The drawing under review shows one solid part. Ordinate dimensions are in mm from its lowest x, y, z. Coordinates: 2 decimals unless noted, no trailing zeros. Write each loop counter-clockwise with the first axis right and the second up, starting at its lowest first coordinate (ties: lowest second). Pieces come first, ordered by that corner, then holes.
Q1. Add section B-B, the plane z = 0.3. Give the number of separate pieces and of enclosed holes in the cut face, plus the area to 3 significant figures.
Q2. To check wall thickness, follow probe 1 along Y at (x, z) = (40, 0.2); probe 2 along Y at (x, z) = (34, 0.85) (1 decimal); probe 3 along X at (y, z) = (15, 0.5) (1 decimal). State the ranges of each line that lie inside material, in increasing order.
Q3. Add section A-A, the plane y = 40. Give the boundary of the cut face in (x, z).
Q4. Add section D-D, the plane y = 62.5. Give the boundary of the cut face in (x, z).
Q5. Add section C-C, the plane x = 40. Give the boundary of the cut face in (y, z).
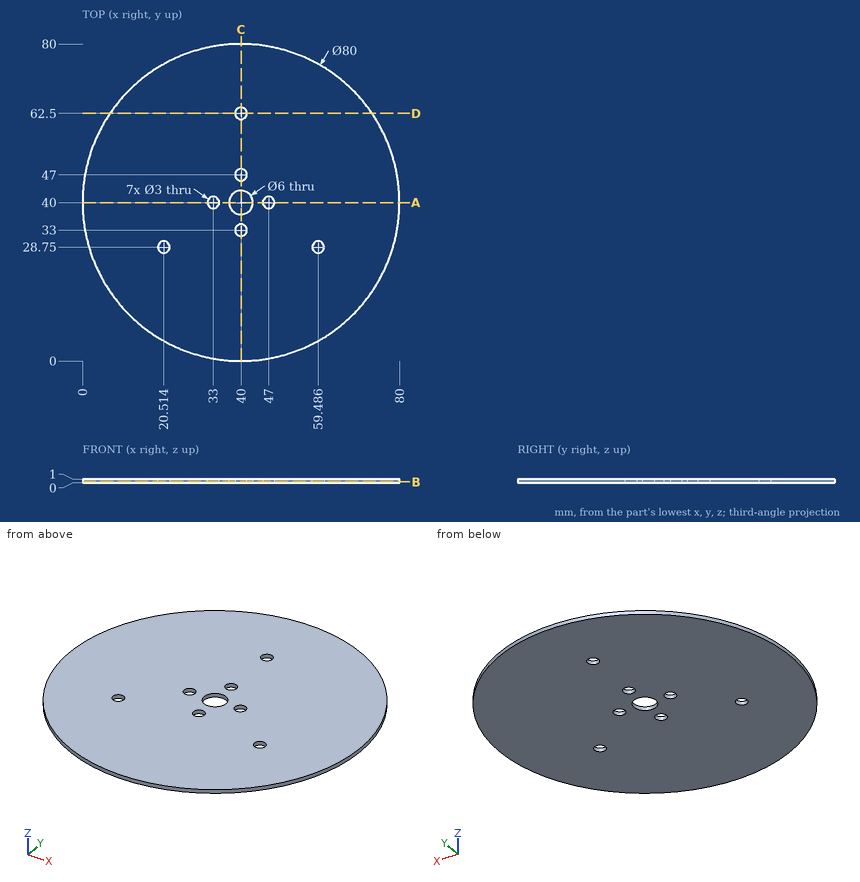
Here are the results:
1. separate pieces: 1
1. enclosed holes: 8
1. area: 4,950 mm2
2. probe 1: y = 0 to 31.5, 34.5 to 37, 43 to 45.5, 48.5 to 61, 64 to 80
2. probe 2: y = 0.5 to 38.9, 41.1 to 79.5
2. probe 3: x = 8.8 to 71.2
3. outline: (0, 0) - (31.5, 0) - (31.5, 1) - (0, 1) - close; (34.5, 0) - (37, 0) - (37, 1) - (34.5, 1) - close; (43, 0) - (45.5, 0) - (45.5, 1) - (43, 1) - close; (48.5, 0) - (80, 0) - (80, 1) - (48.5, 1) - close
4. outline: (6.93, 0) - (38.5, 0) - (38.5, 1) - (6.93, 1) - close; (41.5, 0) - (73.07, 0) - (73.07, 1) - (41.5, 1) - close
5. outline: (0, 0) - (31.5, 0) - (31.5, 1) - (0, 1) - close; (34.5, 0) - (37, 0) - (37, 1) - (34.5, 1) - close; (43, 0) - (45.5, 0) - (45.5, 1) - (43, 1) - close; (48.5, 0) - (61, 0) - (61, 1) - (48.5, 1) - close; (64, 0) - (80, 0) - (80, 1) - (64, 1) - close
